Print and shaded views of the part. All mm, measured from the part's lowest x, y and z. A direction names the side the tool comes from. Coordinates: 2 decimals unless noted, no trailing zeros. Write item = value, one per line.
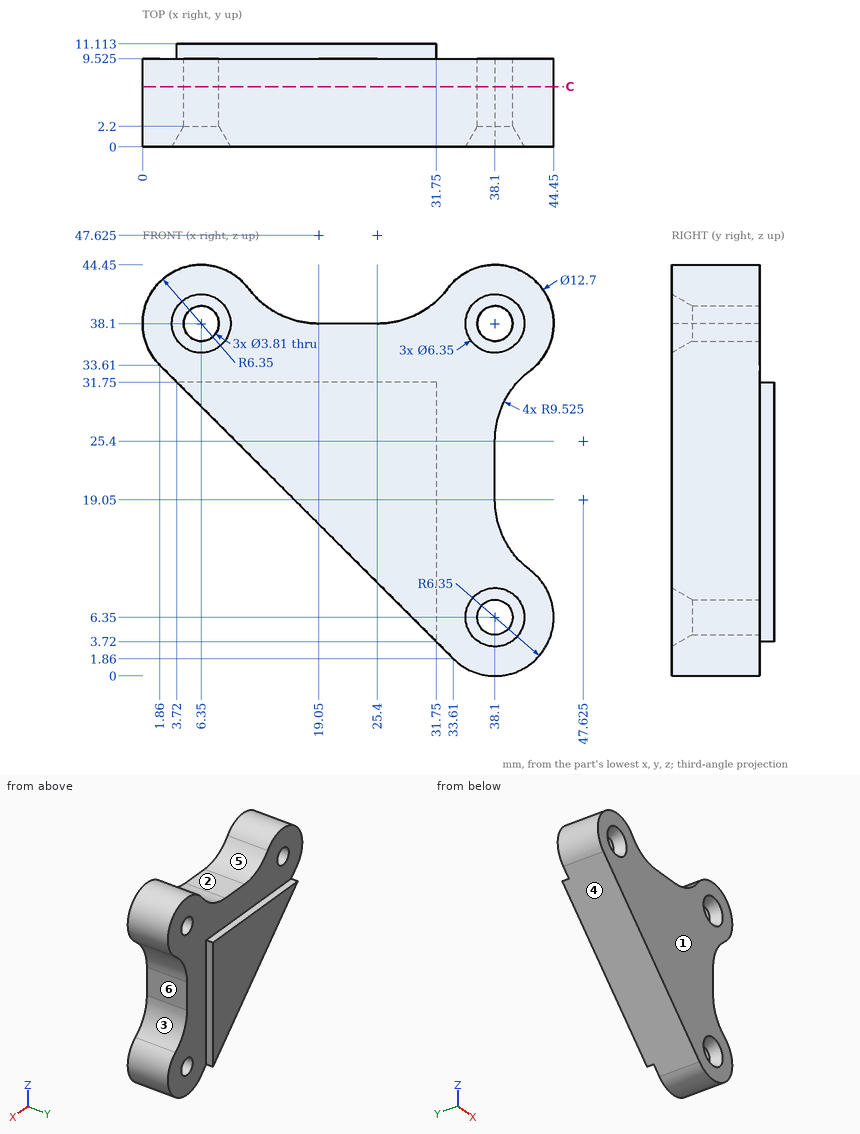
Q1. Saw through at C-C on y = 6.5. Count the separate pieces of the cut face and the enclosed holes in it, and give its area (3 significant figures).
Model answer:
separate_pieces = 1
enclosed_holes = 3
area = 1,030 mm²
Q2. Probe line 1 (X direction, y = 2.25, z = 38); line 2 (Y direction, x = 32.5, z = 4) (1 decimal); line 3 (X direction, y = 1, z = 39.5) (1 decimal). List the from-to ranges inside material, lowest first. Write a range as from..to.
Model answer:
line_1 = 0..4.45, 8.25..36.2, 40..44.45
line_2 = 0..9.5
line_3 = 0.2..4.2, 8.5..14.1, 30.4..35.9, 40.3..44.3
Q3. Mould opens along X. For the marked faces 4, 5 and 6 say: released by +X, released by -X, zero draft, split by the parting line, or undercut.
Model answer:
face_4 = released by -X
face_5 = undercut
face_6 = released by +X
Q4. Which spindle directions (+Z, -Z, +X, -X, +Y, -Y) get a long thin tool onto all of the face, cutting with end or side? Do the marked faces 1, 2 and 3. Say none if no direction does.
Model answer:
face_1 = +Z, -Z, +X, -X, -Y
face_2 = +Z, +Y, -Y
face_3 = +X, +Y, -Y
Q5. Pin check, flat tips, straight feed: pin 1 (6 mm diameter, centred on y = 3, z = 32.5, fed in from -X); pin 2 (5 mm diameter, centred on x = 38.1, z = 38.1, fed in from -Y); pin 3 (6 mm diameter, centred on x = 6.35, z = 38.1, fed in from -Y) (1 decimal); pin 4 (1.5 mm diameter, centred on x = 15, z = 35.5, fed in from -Y). Stop position of each tip, or through.
Model answer:
pin_1 = 0.56
pin_2 = 1.17
pin_3 = 0.3
pin_4 = 0
